Autodesk Inventor part; units mm, degrees
ref_plane "YZ Plane" through (0, 0, 0) normal (1, 0, 0) x (0, 1, 0)
ref_plane "XZ Plane" through (0, 0, 0) normal (0, 1, 0) x (-1, 0, 0)
ref_plane "XY Plane" through (0, 0, 0) normal (0, 0, 1) x (1, 0, 0)
sketch "Sketch1" plane through (0, 0, 0) normal (0, 0, 1) x (1, 0, 0)
  circle A0 centre (0, 0) radius 6.35
  circle A1 centre (0, 0) radius 3.175
  circle A2 centre (0, 0) radius 0.9922
  dimension "d0" = 12.7
  dimension "d1" = 6.35
  dimension "d2" = 1.9844
extrude "Extrusion1" add sketch "Sketch1" along normal blind 2.032 contours A0 | A1
extrude "Extrusion2" add sketch "Sketch1" against normal blind 3.302 contours A1
sketch "Sketch2" plane through (0, 0, 0) normal (1, 0, 0) x (0, 1, 0)
  circle A0 centre (0, -1.651) radius 0.7112
  line L0 (-3.175, -3.302) -> (3.175, -3.302)
  point P0 (0, 0)
  dimension "d7" = 1.4224
  dimension "d8" = 1.651
extrude "Extrusion3" cut sketch "Sketch2" against normal blind 3.302
properties part number "Flywheel"
Could you check a few things on this model? Use its own coordinates, in mm. A direction names the side the tool comes from. Give positions to 0.01 mm unless a question says otherwise; leave off trailing zeros. Order: outer loops, then holes, each group sorted by start corner. A loop starts at its lowest first (then second) coordinate and runs counter-clockwise, first axis right, second up. Notation, with made-up numbers: M -31,3.5 L 9,3.5 A11 ccw 9,19.5 Z; hole C 58,-7.5 d6. An arc over 180 degrees is marked long. One line per question, with ' | ' between items.
1. For faces 1 (the face through (-1.92, 0.66, -1.92)), 2 (the face through (-1.38, 6.2, 1)), 3 (the face through (-2, 3, 0)), which set-ups out of +Z, -Z, +X, -X, +Y, -Y let a thin tool reach every point of the face, with its end or its side?
Results:
face 1: -X | face 2: +Z, -Z | face 3: -Z
2. We'd pull the mould along Y, two halves only. Please class faces 4 (the face through (0.917, -0.38, -0.598)), 5 (the face through (3.03, 0.95, -1.63)), 6 (the face through (1.3, 0.1, 2.032)): +Y half, -Y half, draft (parallel to the pull), parting line (faces both ways), or undercut.
Results:
face 4: undercut | face 5: parting line | face 6: draft
3. I want a section at A-A (x = 0). List the corners of the cut face in (y, z) for me (3 decimals), and give its area (3 significant figures).
Results:
outline: M -6.35,0 L -3.175,0 L -3.175,-3.302 L -0.992,-3.302 L -0.992,2.032 L -6.35,2.032 Z; M 0.992,-3.302 L 3.175,-3.302 L 3.175,0 L 6.35,0 L 6.35,2.032 L 0.992,2.032 Z | area: 36.2 mm²
4. If I drill on line 1 (Y direction, x = 0, z = -0.7) (3 decimals); line 2 (Z direction, x = 4.5, y = -2), over which ranges is the centre line in solid material (lowest first)?
Results:
line 1: -3.175 to -0.992, 0.992 to 3.175 | line 2: 0 to 2.03
5. I want a section at C-C (z = -2.55). List the corners of the cut face in (x, y) for me (3 decimals).
Results:
outline: C 0,0 d6.35; hole C 0,0 d1.984
6. I want a section at D-D (y = 1.75). List the corners of the cut face in (x, z) for me.
Results:
outline: M -6.1,0 L -2.65,0 L -2.65,-3.3 L 2.65,-3.3 L 2.65,0 L 6.1,0 L 6.1,2.03 L -6.1,2.03 Z
7. I want a section at B-B (y = 0). List the corners of the cut face in (x, z) for me (3 decimals).
Results:
outline: M -6.35,0 L -3.175,0 L -3.175,-0.94 L -0.992,-0.94 L -0.992,2.032 L -6.35,2.032 Z; M -3.175,-3.302 L -0.992,-3.302 L -0.992,-2.362 L -3.175,-2.362 Z; M 0.992,-3.302 L 3.175,-3.302 L 3.175,0 L 6.35,0 L 6.35,2.032 L 0.992,2.032 Z
8. I'm going to push flat-ended pins straight in: pin 1 (3 mm diameter, centred on y = 5, z = 0, fed in from -X); pin 2 (3 mm diameter, centred on y = -1.5, z = -2, fed in from -X); pin 3 (1.6 mm diameter, centred on x = 0, y = 0, fed in from -Z); pin 4 (2.5 mm diameter, centred on y = 0, z = -1.651, fed in from +X) (3 decimals). Where does each tip first touch, or does it pass through?
Results:
pin 1: x = -5.3 | pin 2: x = -3.17 | pin 3: through | pin 4: x = 3.175
